Here's how the part is built. I have some questions about the finished solid (model axes, mm). Face numbers are marked on the shaded views. A direction names the side the tool comes from. Give positions to 0.01 mm unless a question says otherwise; leave off trailing zeros. Write each loop counter-clockwise with the first axis right and the second up, starting at its lowest first coordinate (ties: lowest second). Pieces come first, ordered by that corner, then holes. Notation, with made-up numbers: (-28.75, 82) - (8.25, 82) arc R18 cw to (8.25, 114) - close; hole circle Ø5 at (51, 62). An arc over 180 degrees is marked (long way). Use one line per item in the form item = value. Start each with the question number.
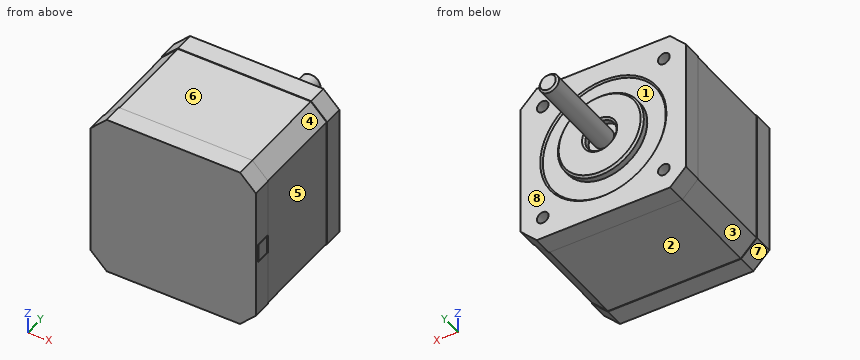
from build123d import *

# Parameters (mm, degrees)
SKETCH1_W           = 42
SKETCH1_H           = 42
BOSS_EXTRUDE1_DEPTH = 34
CHAMFER1_SIZE       = 4
BOSS_EXTRUDE4_DEPTH = 5
BOSS_EXTRUDE5_DEPTH = 5
SKETCH2_R           = 16.25
CUT_EXTRUDE1_DEPTH  = 0.4
SKETCH3_R           = 11
SKETCH3_R_2         = 4
BOSS_EXTRUDE2_DEPTH = 1.9
SKETCH4_R           = 2.5
BOSS_EXTRUDE3_DEPTH = 23
CHAMFER2_SIZE       = 0.5
SKETCH5_R           = 1.5
CUT_EXTRUDE2_DEPTH  = 5
SKETCH8_W           = 4.8
SKETCH8_H           = 3.8
SKETCH8_W_2         = 4.5
SKETCH8_H_2         = 3.5
BOSS_EXTRUDE6_DEPTH = 0.1


with BuildPart() as part:
    # Sketch1 → Boss-Extrude1 (new body)
    with BuildSketch(Plane(origin=(0, 0, 0), x_dir=(1, 0, 0), z_dir=(0, 1, 0))):
        Rectangle(SKETCH1_W, SKETCH1_H)
    extrude(amount=BOSS_EXTRUDE1_DEPTH)

    # Chamfer1
    chamfer1_edges = [part.edges().sort_by_distance(p)[0] for p in [
        (21, 17, 21),
        (-21, 17, 21),
        (-21, 17, -21),
        (21, 17, -21),
    ]]
    chamfer(chamfer1_edges, length=CHAMFER1_SIZE)

    # Sketch6 → Boss-Extrude4 (add)
    with BuildSketch(Plane(origin=(0, 34, 0), x_dir=(1, 0, 0), z_dir=(0, 1, 0))):
        Polygon((17.062132034, 21.15), (-17.062132034, 21.15), (-21.15, 17.062132034), (-21.15, -17.062132034), (-17.062132034, -21.15), (17.062132034, -21.15), (21.15, -17.062132034), (21.15, 17.062132034), align=None)
    extrude(amount=-BOSS_EXTRUDE4_DEPTH)

    # Sketch7 → Boss-Extrude5 (add)
    with BuildSketch(Plane.XZ):
        Polygon((-21.15, 17.062132034), (-21.15, -17.062132034), (-17.062132034, -21.15), (17.062132034, -21.15), (21.15, -17.062132034), (21.15, 17.062132034), (17.062132034, 21.15), (-17.062132034, 21.15), align=None)
    extrude(amount=-BOSS_EXTRUDE5_DEPTH)

    # Sketch2 → Cut-Extrude1 (cut)
    with BuildSketch(Plane(origin=(0, 34, 0), x_dir=(1, 0, 0), z_dir=(0, 1, 0))):
        with Locations(Location((0, 0, 0), (0, 0, 270))):
            Circle(SKETCH2_R)
    extrude(amount=-CUT_EXTRUDE1_DEPTH, mode=Mode.SUBTRACT)

    # Sketch3 → Boss-Extrude2 (add)
    with BuildSketch(Plane(origin=(0, 33.6, 0), x_dir=(1, 0, 0), z_dir=(0, 1, 0))):
        with Locations(Location((0, 0, 0), (0, 0, 90))):
            Circle(SKETCH3_R)
        with Locations(Location((0, 0, 0), (0, 0, 90))):
            Circle(SKETCH3_R_2, mode=Mode.SUBTRACT)
    extrude(amount=BOSS_EXTRUDE2_DEPTH)

    # Sketch4 → Boss-Extrude3 (add)
    with BuildSketch(Plane(origin=(0, 33.6, 0), x_dir=(1, 0, 0), z_dir=(0, 1, 0))):
        with Locations(Location((0, 0, 0), (0, 0, 270))):
            Circle(SKETCH4_R)
    extrude(amount=BOSS_EXTRUDE3_DEPTH)

    # Chamfer2
    # the kernel refuses this chamfer: 0.5 mm, written as the material it adds along each edge
    with BuildSketch(Plane(origin=(0, 33.6, 0), x_dir=(0, 0, 1), z_dir=(-1, 0, 0))) as chamfer2_piece_1_section:
        Polygon((16.25, CHAMFER2_SIZE), (16.25 - CHAMFER2_SIZE, 0), (16.25, 0), align=None)
    chamfer2_piece_1 = revolve(axis=Axis((0, 33.6, 0), (0, 1, 0)), mode=Mode.PRIVATE)
    chamfer2_piece_1 = split(chamfer2_piece_1, bisect_by=Plane(origin=(0, 34, -15.959627936), z_dir=(0, -1, 0)), keep=Keep.TOP, mode=Mode.PRIVATE)
    add(chamfer2_piece_1)
    # the kernel refuses this chamfer: 0.5 mm, written as the material it takes off along each edge
    with BuildSketch(Plane(origin=(0, 35.5, 0), x_dir=(0, 0, -1), z_dir=(1, 0, 0))) as chamfer2_2_piece_1:
        Polygon((4 + CHAMFER2_SIZE, 0), (4, -CHAMFER2_SIZE), (4, 0), align=None)
    revolve(axis=Axis((0, 35.5, 0), (0, 1, 0)), mode=Mode.SUBTRACT)
    with BuildSketch(Plane(origin=(0, 35.5, 0), x_dir=(0, 0, -1), z_dir=(1, 0, 0))) as chamfer2_2_piece_2:
        Polygon((11, -CHAMFER2_SIZE), (11 - CHAMFER2_SIZE, 0), (11, 0), align=None)
    revolve(axis=Axis((0, 35.5, 0), (0, 1, 0)), mode=Mode.SUBTRACT)
    with BuildSketch(Plane(origin=(0, 56.6, 0), x_dir=(0, 0, 1), z_dir=(-1, 0, 0))) as chamfer2_2_piece_3:
        Polygon((2.5, -CHAMFER2_SIZE), (2.5 - CHAMFER2_SIZE, 0), (2.5, 0), align=None)
    revolve(axis=Axis((0, 56.6, 0), (0, 1, 0)), mode=Mode.SUBTRACT)

    # Sketch5 → Cut-Extrude2 (cut)
    with BuildSketch(Plane(origin=(0, 34, 0), x_dir=(1, 0, 0), z_dir=(0, 1, 0))):
        with Locations(Location((-15.5, 15.5, 0), (0, 0, 270))):
            Circle(SKETCH5_R)
        with Locations(Location((15.5, 15.5, 0), (0, 0, 270))):
            Circle(SKETCH5_R)
        with Locations(Location((15.5, -15.5, 0), (0, 0, 270))):
            Circle(SKETCH5_R)
        with Locations(Location((-15.5, -15.5, 0), (0, 0, 270))):
            Circle(SKETCH5_R)
    extrude(amount=-CUT_EXTRUDE2_DEPTH, mode=Mode.SUBTRACT)

    # Sketch8 → Boss-Extrude6 (add)
    with BuildSketch(Plane(origin=(21.15, 0, 0), x_dir=(0, 0, -1), z_dir=(1, 0, 0))):
        with Locations((0.269797982, 2.75)):
            Rectangle(SKETCH8_W, SKETCH8_H)
        with Locations((0.269797982, 2.75)):
            Rectangle(SKETCH8_W_2, SKETCH8_H_2, mode=Mode.SUBTRACT)
    extrude(amount=BOSS_EXTRUDE6_DEPTH)


solid = part.part
1. We'd pull the mould along Y, two halves only. Please class the marked faces 6, 7 and 8: pulls with the +Y half, pulls with the -Y half, needs draft (parallel to the pull), parting line crosses it, or undercut.
2. I want a section at A-A, the plane y = 14. List the corners of the cut face in (x, z) for me.
3. For P1, Ø2.5, axis at x = 15.5, z = -15.5, coming from the +Y side; P2, Ø6, axis at y = 42.5, z = -2, coming from the -X side; P3, Ø5, axis at x = -7.5, z = -13.5, coming from the +Y side, each with a flat end and sliding along its axis, tell me the tip position at first contact or that it passes through.
4. Please list where these lines run through material, in increasing order: line 1 (X direction, y = 32.4, z = 15.5); line 2 (X direction, y = 31.5, z = -15).
5. I want a section at B-B, the plane y = 51. List the corners of the cut face in (x, z) for me.
6. For the marked faces 1, 2, 3, 4 and 5, which set-ups out of +Z, -Z, +X, -X, +Y, -Y let a thin tool reach every point of the face, with its end or its side?
Result sheet:
q1.face_6 = undercut
q1.face_7 = needs draft
q1.face_8 = pulls with the +Y half
q2.outline = (-21, -17) - (-17, -21) - (17, -21) - (21, -17) - (21, 17) - (17, 21) - (-17, 21) - (-21, 17) - close
q3.P1 = 29
q3.P2 = -2.5
q3.P3 = 34
q4.line_1 = -21.15 to -17, -14 to 14, 17 to 21.15
q4.line_2 = -21.15 to -16.91, -14.09 to 14.09, 16.91 to 21.15
q5.outline = circle Ø5 at (0, 0)
q6.face_1 = +Y
q6.face_2 = -Z, +X, -X
q6.face_3 = -Z, -X
q6.face_4 = +Z, +X
q6.face_5 = +Z, -Z, +X
